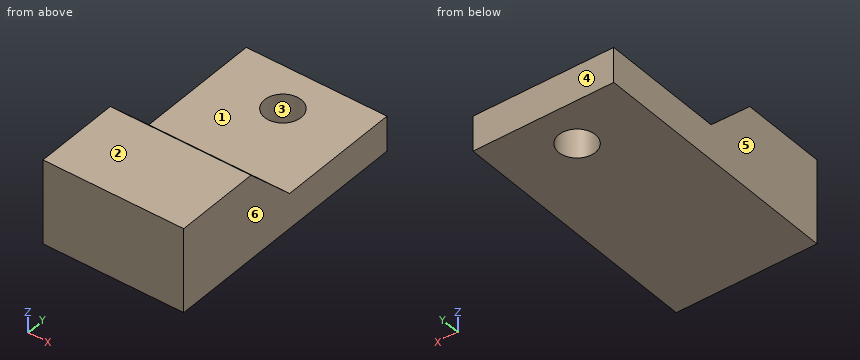
```python
from build123d import *

# Parameters (mm, degrees)
SKICA1_W                = 20
SKICA1_H                = 36.830083089
SKICA1_R                = 2.6
P_IDAT_VYSUNUT_M1_DEPTH = 5
SKICA2_W                = 20
SKICA2_H                = 19.184386705
P_IDAT_VYSUNUT_M2_DEPTH = 7
ZKOSEN_1_SIZE           = 7


with BuildPart() as part:
    # Skica1 → Přidat vysunutím1 (new body)
    with BuildSketch(Plane.XY):
        with Locations((14.524287798, -297.284958456)):
            Rectangle(SKICA1_W, SKICA1_H)
        with Locations((14.524287798, -284.981509323)):
            Circle(SKICA1_R, mode=Mode.SUBTRACT)
    extrude(amount=P_IDAT_VYSUNUT_M1_DEPTH)

    # Skica2 → Přidat vysunutím2 (add)
    with BuildSketch(Plane.XY.offset(5)):
        with Locations((14.524287798, -306.107806648)):
            Rectangle(SKICA2_W, SKICA2_H)
    extrude(amount=P_IDAT_VYSUNUT_M2_DEPTH)

    # Zkosení1
    zkosen_1_edges = [part.edges().sort_by_distance(p)[0] for p in [
        (14.524287798, -296.515613295, 12),
    ]]
    chamfer(zkosen_1_edges, length=ZKOSEN_1_SIZE - 0.0001)  # a hair under: the kernel refuses the full size


solid = part.part
```
Check sheet for the modelled part. Datum: model origin and axes. Units: mm. Face numbers are marked on the shaded views. A direction names the side the tool comes from. Coordinates: 2 decimals unless noted, no trailing zeros. Loops run counter-clockwise (first coordinate to the right, second up) from the corner with the lowest first, then second, coordinate; pieces in that order, holes last.
1) Release check for a two-part mould opening along X. For the marked faces 3, 4, 5 and 6 record: released by +X, released by -X, zero draft, split by the parting line, or undercut.
2) Sectioned sample at A-A (y = -286.5). Record the boundary of the cut face in (x, z), and give its area (3 significant figures).
3) Access from +Z, -Z, +X, -X, +Y, -Y to the whole of each face (thin tool, end or side, straight path). Record for the marked faces 1 and 2.
4) Material ranges on probe 1 along Z at (x, y) = (12.5, -289.5); probe 2 along X at (y, z) = (-284, 0.5); probe 3 along Y at (x, z) = (16.75, 4), recorded low to high.
5) Gauge pin test, flat end, axial feed: pin 1 (7 mm diameter, centred on x = 14.52, y = -284.98, fed in from +Z). Record the tip position at first contact, or that the pin passes through.
6) Sectioned sample at D-D (z = 1.5). Record the boundary of the cut face in (x, y).
Check sheet entries:
1. face 3: undercut
1. face 4: zero draft
1. face 5: released by -X
1. face 6: released by +X
2. outline: (4.52, 0) - (12.41, 0) - (12.41, 5) - (4.52, 5) - close; (16.63, 0) - (24.52, 0) - (24.52, 5) - (16.63, 5) - close
2. area: 78.9 mm2
3. face 1: +Z, +X, -X, +Y
3. face 2: +Z, +X, -X, +Y, -Y
4. probe 1: z = 0 to 5
4. probe 2: x = 4.52 to 12.12, 16.93 to 24.52
4. probe 3: y = -315.7 to -286.33, -283.64 to -278.87
5. pin 1: stops at z = 5
6. outline: (4.52, -315.7) - (24.52, -315.7) - (24.52, -278.87) - (4.52, -278.87) - close; hole circle Ø5.2 at (14.52, -284.98)
